Verification items for this drawing (mm, ordinates from the low corner). Give positions to 0.01 mm unless a question says otherwise; leave off trailing zeros. Loops run counter-clockwise (first coordinate to the right, second up) from the corner with the lowest first, then second, coordinate; pieces in that order, holes last. Notation, with made-up numbers: (-21, 23) -> (14, 23) arc R23 cw to (14, 53) -> close; hole circle Ø5 at (-29, -40). An arc over 180 degrees is marked (long way). Write each question's results on one line, items separated by ' | '. Start each with the question number.
Item 1: Cross-section at D-D on y = 16.5. Enter the section's corners in (x, z).
Item 2: Mould release check, pull along X, two halves, no side actions. Record for the marked faces 1, 2, 3 and 4: pulls with the +X half, pulls with the -X half, needs draft (parallel to the pull), parting line crosses it, or undercut.
Item 3: Gauge pin test, flat end, axial feed: pin 1 Ø2.5 at (x, y) = (3.5, 10) entering from -Z. Record the tip position at first contact, or that the pin passes through.
Item 4: Cross-section at B-B on y = 10. Enter the section's corners in (x, z), then the cut area to 3 significant figures.
Item 5: Scan lines: line 1 along Y through (x, z) = (15, 0.65); line 2 along Y through (x, z) = (3.5, 4.25); line 3 along Z through (x, y) = (20.5, 15). Record each from-to range of solid material in increasing order.
Item 6: Cross-section at C-C on z = 6. Enter the section's corners in (x, y).
Item 7: Cross-section at A-A on x = 26.5. Enter the section's corners in (y, z), then the cut area to 3 significant figures.
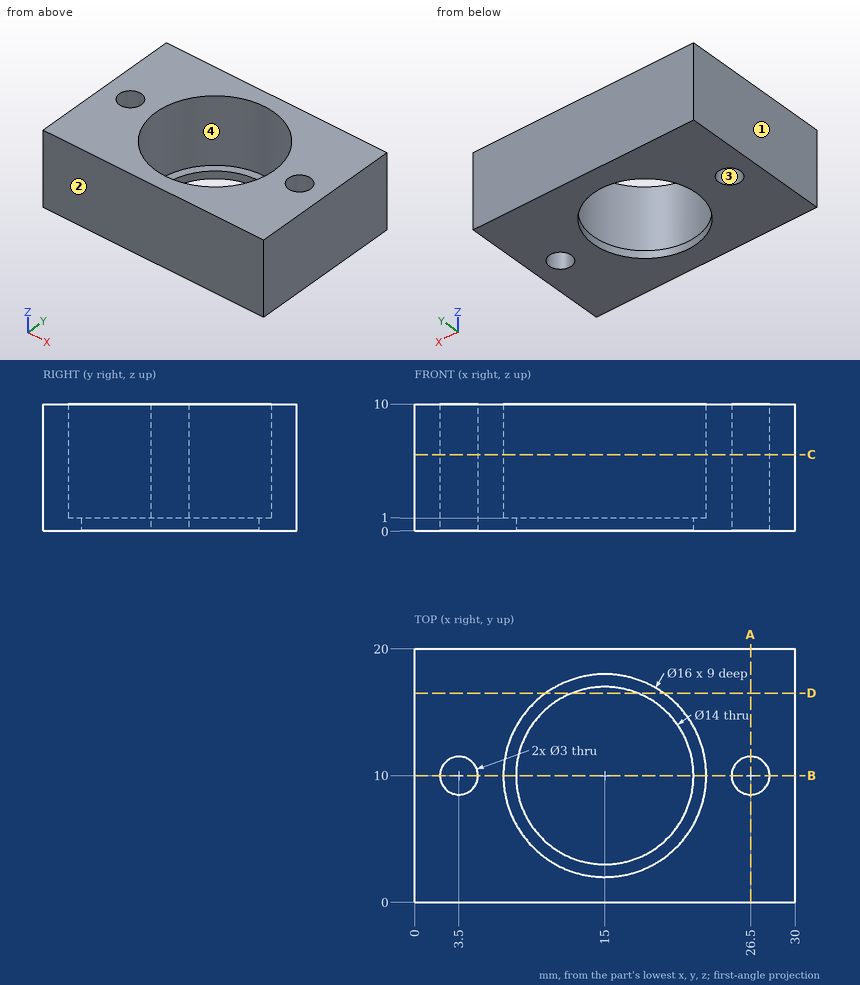
Answer sheet:
1) outline: (0, 0) -> (12.4, 0) -> (12.4, 1) -> (10.34, 1) -> (10.34, 10) -> (0, 10) -> close; (17.6, 0) -> (30, 0) -> (30, 10) -> (19.66, 10) -> (19.66, 1) -> (17.6, 1) -> close
2) face 1: pulls with the -X half | face 2: needs draft | face 3: undercut | face 4: undercut
3) pin 1: passes through
4) outline: (0, 0) -> (2, 0) -> (2, 10) -> (0, 10) -> close; (5, 0) -> (8, 0) -> (8, 1) -> (7, 1) -> (7, 10) -> (5, 10) -> close; (22, 0) -> (25, 0) -> (25, 10) -> (23, 10) -> (23, 1) -> (22, 1) -> close; (28, 0) -> (30, 0) -> (30, 10) -> (28, 10) -> close | area: 82.0 mm²
5) line 1: y = 0 to 3, 17 to 20 | line 2: y = 0 to 8.5, 11.5 to 20 | line 3: z = 0 to 1
6) outline: (0, 0) -> (30, 0) -> (30, 20) -> (0, 20) -> close; hole circle Ø3 at (3.5, 10); hole circle Ø16 at (15, 10); hole circle Ø3 at (26.5, 10)
7) outline: (0, 0) -> (8.5, 0) -> (8.5, 10) -> (0, 10) -> close; (11.5, 0) -> (20, 0) -> (20, 10) -> (11.5, 10) -> close | area: 170 mm²
